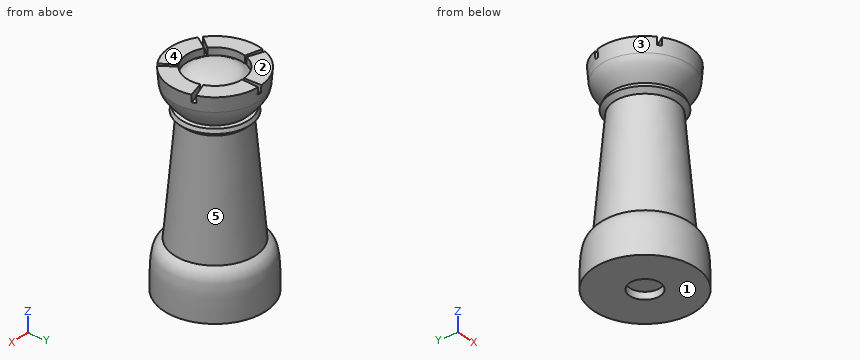
Autodesk Fusion 360 part; units mm, degrees
sketch "Sketch1" plane through (0, 0, 0) normal (0, 1, 0) x (1, 0, 0)
  line L0 (0, 0) -> (0, -70)
  line L1 (0, 0) -> (-17.5, 0)
  spline S0 degree 5 poles (-17.5, 0) (-17.5, -1.949) (-17.4812, -5.4749) (-17.3967, -9.6483) (-17.034, -13.32) (-15.2217, -16.0242) (-11.5143, -17.5778) (-6.6893, -18.7492) (-2.4074, -19.5755) (0, -20) knots 0 0 0 0 0 0 0.2 0.4 0.6 0.8 1 1 1 1 1 1
  line L2 (-5, -19.1184) -> (5, -20.8816)
  line L3 (-17.5, 4) -> (-17.5, -4)
  line L4 (-15.4223, 0) -> (-10.3547, -57.9233)
  spline S1 degree 5 poles (-10.3547, -57.9233) (-10.6938, -58.2624) (-11.3394, -58.9222) (-12.2103, -59.8566) (-13.1936, -61.0089) (-14.1589, -62.3571) (-14.7035, -63.4078) (-14.9524, -64.1982) (-15.0388, -64.7286) (-15.0621, -64.9946) knots 0 0 0 0 0 0 0.2 0.4 0.6 0.8 1 1 1 1 1 1
  line L5 (-15.0621, -64.9946) -> (-15.5, -70)
  line L6 (-14.9783, -64.0369) -> (-15.1459, -65.9522)
  line L7 (-17.5, -70) -> (0, -70) construction
  line L8 (-15.5, -70) -> (-9.7348, -70)
  line L9 (-9.7348, -70) -> (-9.7348, -67.5)
  line L10 (-9.0716, -56.6402) -> (-11.6378, -59.2064)
  line L11 (-17.5, 0) -> (-17.5, -70) construction
  spline S2 degree 5 poles (-9.7348, -67.5) (-9.5938, -67.5) (-9.3202, -67.5511) (-8.9352, -67.7806) (-8.3991, -68.3325) (-7.2315, -69.1675) (-5.359, -69.7194) (-3.0799, -69.9489) (-1.103, -70) (0, -70) knots 0 0 0 0 0 0 0.2 0.4 0.6 0.8 1 1 1 1 1 1
  line L12 (-10.1589, -67.5) -> (-9.3107, -67.5)
  line L13 (-3.3162, -70) -> (3.3162, -70)
  line L14 (-10.3504, -57.9716) -> (-11.575, -57.6845)
  line L15 (-12.1293, -56.3884) -> (-10.6186, -54.9071)
  line L16 (-11.575, -57.6845) -> (-12.1293, -56.3884)
  line L17 (-5.25, 0) -> (-5.25, -2.5)
  line L18 (-5.25, -2.5) -> (0, -2.5)
  dimension "d1" = 70
  dimension "d2" = 17.5
  dimension "d3" = 5
  dimension "d4" = 45
  dimension "d5" = 5
  dimension "d6" = 10
  dimension "d14" = 2.5
  dimension "d15" = 2
  dimension "d16" = 2.5
  dimension "d17" = 5.25
revolve "Revolve1" add sketch "Sketch1" angle 360 about axis through (0, 0, 0) along (0, 0, 1) contours L0 L1 S0 L4 L17 L18 | L0 S0 L4 S1 L5 L6 L8 L9 L10 S2 | L1 S0 L4 | L4 S1 L10 L14 L15 L16
sketch "Sketch3" plane through (0, 0, 70) normal (0, 0, 1) x (-1, 0, 0)
  circle A0 centre (0, 0) radius 9.7348
  circle A1 centre (0, 0) radius 15.5
  line L0 (0, 0) -> (0.6761, -15.4852)
  line L1 (0, 0) -> (-0.6761, -15.4852)
  line L2 (0, 0) -> (0, -15.5) construction
  dimension "d8" = 5
  dimension "d9" = 2.5
extrude "Extrude1" cut sketch "Sketch3" against normal up to surface (2.5 mm away) contours A0 A1 L0 L1 picked at (0.4421, -13.5697)
pattern_circular "C-Pattern1" count 5 over 360 about axis through (0, 0, 1.75) along (0, 0, 1) of "Extrude1"
equation "d2 = 3.5 cm / 2"
Check sheet for the modelled part. Datum: model origin and axes. Units: mm. Face numbers are marked on the shaded views. A direction names the side the tool comes from. Round coordinates to 2 decimals unless told otherwise and drop trailing zeros. Order: outer loops, then holes, each group sorted by start corner. A loop starts at its lowest first (then second) coordinate and runs counter-clockwise, first axis right, second up. Notation, with made-up numbers: (81, 6.5) -> (113, 6.5) arc R23 ccw to (113, 37.5) -> close; hole circle Ø9 at (4, -26.5). An arc over 180 degrees is marked (long way). One line per item, written item: value. Start each with the question number.
Q1. Cross-section at A-A (z = 44). Record the boundary of the cut face in (x, y).
Q2. Mould release check, pull along Z, two halves, no side actions. Record for the marked faces 1, 2 and 3: pulls with the +Z half, pulls with the -Z half, needs draft (parallel to the pull), parting line crosses it, or undercut.
Q3. Cross-section at B-B (z = 32). Record the boundary of the cut face in (x, y).
Q4. Gauge pin test, flat ends, axial feed: pin 1 Ø12 at (x, y) = (6.5, -5.5) entering from -Z; pin 2 Ø4 at (x, z) = (-13.5, 18) entering from -Y; pin 3 Ø6 at (y, z) = (-3.5, 58.5) entering from -X; pin 4 Ø5 at (x, z) = (-7.5, 26) entering from +Y. Record the tip position at first contact, or that the pin passes through.
Q5. Thickness scan on line 1 (Y direction, x = 0, z = 0.5); line 2 (Y direction, x = 8.5, z = 28.5). Record the ranges inside material, lowest first.
Q6. Set-up check for the marked faces 4 and 5: record each of +Z, -Z, +X, -X, +Y, -Y from which the full face is reachable in a straight line by a thin tool's end or side.
Completed:
1. outline: circle Ø23.15 at (0, 0)
2. face 1: pulls with the -Z half
2. face 2: pulls with the +Z half
2. face 3: undercut
3. outline: circle Ø25.25 at (0, 0)
4. pin 1: stops at z = 0
4. pin 2: stops at y = -7.73
4. pin 3: stops at x = -13.16
4. pin 4: stops at y = 12.19
5. line 1: y = -17.5 to -5.25, 5.25 to 17.5
5. line 2: y = -9.74 to 9.74
6. face 4: +Z, +X, -X, +Y, -Y
6. face 5: none
